Source: three-view drawing plus pictorial views. Frame: mm from the lowest corner of the part. A direction names the side the tool comes from. Give positions to 0.01 mm unless a question says otherwise; leave off trailing zeros. Loops run counter-clockwise (first coordinate to the right, second up) from the corner with the lowest first, then second, coordinate; pieces in that order, holes last. Notation, with made-up numbers: (-25.5, 86.25) - (-11.5, 86.25) arc R7 ccw to (-11.5, 92.25) - close; hole circle Ø3 at (68, 15). An arc over 180 degrees is marked (long way). Answer as a JSON object with one key per item and string values.
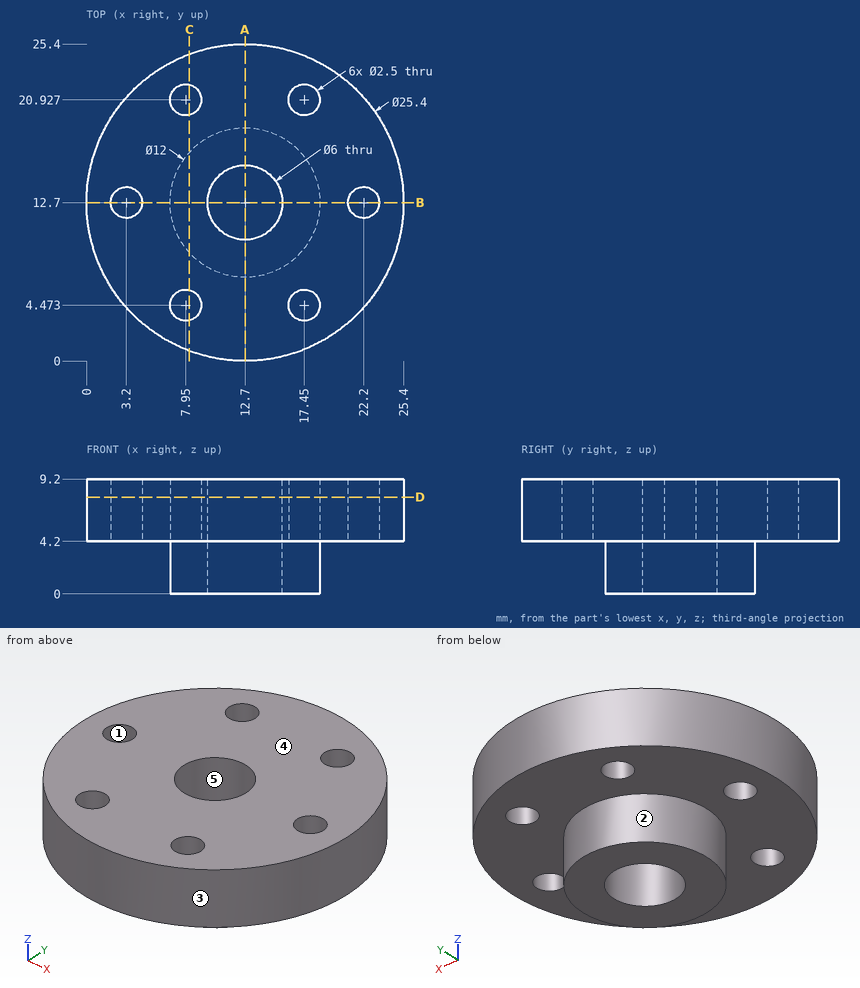
Item 1: Cut plane A-A (x = 12.7). Return loops of the section in (y, z), then the cut area to 3 significant figures.
Geometry check:
{"outline": "(0, 4.2) - (6.7, 4.2) - (6.7, 0) - (9.7, 0) - (9.7, 9.2) - (0, 9.2) - close; (15.7, 0) - (18.7, 0) - (18.7, 4.2) - (25.4, 4.2) - (25.4, 9.2) - (15.7, 9.2) - close", "area": "122 mm2"}
Item 2: Material intervals for line 1 (X direction, y = 22, z = 7.25); line 2 (Y direction, x = 8, z = 8); line 3 (Y direction, x = 16.5, z = 6.5) (1 decimal), sorted ascending. Write a range as [from, to].
Geometry check:
{"line 1": "x = [4.05, 7.31], [8.59, 16.81], [18.09, 21.35]", "line 2": "y = [0.9, 3.22], [5.72, 19.68], [22.18, 24.5]", "line 3": "y = [0.6, 3.7], [5.3, 20.1], [21.7, 24.8]"}
Item 3: Cut plane D-D (z = 7.75). Return loops of the section in (x, y), then the cut area to 3 significant figures.
Geometry check:
{"outline": "circle Ø25.4 at (12.7, 12.7); hole circle Ø2.5 at (3.2, 12.7); hole circle Ø2.5 at (7.95, 4.47); hole circle Ø2.5 at (7.95, 20.93); hole circle Ø6 at (12.7, 12.7); hole circle Ø2.5 at (17.45, 4.47); hole circle Ø2.5 at (17.45, 20.93); hole circle Ø2.5 at (22.2, 12.7)", "area": "449 mm2"}
Item 4: Cut plane B-B (y = 12.7). Return loops of the section in (x, z).
Geometry check:
{"outline": "(0, 4.2) - (1.95, 4.2) - (1.95, 9.2) - (0, 9.2) - close; (4.45, 4.2) - (6.7, 4.2) - (6.7, 0) - (9.7, 0) - (9.7, 9.2) - (4.45, 9.2) - close; (15.7, 0) - (18.7, 0) - (18.7, 4.2) - (20.95, 4.2) - (20.95, 9.2) - (15.7, 9.2) - close; (23.45, 4.2) - (25.4, 4.2) - (25.4, 9.2) - (23.45, 9.2) - close"}
Item 5: Contact query for flat-ended pins moving along their axis: P1, Ø5, axis at x = 21.5, y = 7.5, coming from the -Z side; P2, Ø1.5, axis at y = 14, z = 7.5, coming from the -X side; P3, Ø5, axis at x = 5, z = 1, coming from the -Y side. Output: stop coordinate, or through.
Geometry check:
{"P1": "stops at z = 4.2", "P2": "stops at x = 0.01", "P3": "stops at y = 9.71"}
Item 6: Access query for the marked faces 1 and 2. Directions: +Z, -Z, +X, -X, +Y, -Y. A direction counts if a zero-diameter tool reaches every point of the face in a straight line with its end or side. Return the directions, or none.
Geometry check:
{"face 1": "+Z, -Z", "face 2": "-Z"}
Item 7: Mould query, pull axis Y, two halves, no side actions, for the marked faces 3, 4 and 5. Classes: released by +Y, released by -Y, zero draft, split by the parting line, or undercut.
Geometry check:
{"face 3": "split by the parting line", "face 4": "zero draft", "face 5": "undercut"}
Item 8: Cut plane C-C (x = 8.25). Return loops of the section in (y, z) (1 decimal).
Geometry check:
{"outline": "(0.8, 4.2) - (3.3, 4.2) - (3.3, 9.2) - (0.8, 9.2) - close; (5.7, 4.2) - (8.7, 4.2) - (8.7, 0) - (16.7, 0) - (16.7, 4.2) - (19.7, 4.2) - (19.7, 9.2) - (5.7, 9.2) - close; (22.1, 4.2) - (24.6, 4.2) - (24.6, 9.2) - (22.1, 9.2) - close"}
